from build123d import *

# Parameters (mm, degrees)
SKETCH_1_R      = 16.2
SKETCH_1_R_2    = 14.6
EXTRUDE_1_DEPTH = 2.5
SKETCH_3_R      = 1
FILLET_1_R      = 1


with BuildPart() as part:
    # 草图1 → 凸台-拉伸1 (new body, symmetric)
    with BuildSketch(Plane.XY):
        Circle(SKETCH_1_R)
        Circle(SKETCH_1_R_2, mode=Mode.SUBTRACT)
    extrude(amount=EXTRUDE_1_DEPTH, both=True)

    # 草图3 → 切除-旋转1 (revolve, cut)
    with BuildSketch(Plane(origin=(0, 0, 0), x_dir=(1, 0, 0), z_dir=(0, 1, 0))):
        with Locations((-14.1, 0)):
            Circle(SKETCH_3_R)
    revolve(axis=Axis((0, 0, 2.5), (0, 0, -1)), mode=Mode.SUBTRACT)

    # 圆角1
    fillet_1_edges = [part.edges().sort_by_distance(p)[0] for p in [
        (0, 14.6, 0.866025404),
        (0, -14.6, -0.866025404),
    ]]
    fillet(fillet_1_edges, radius=FILLET_1_R)


solid = part.part
For this review, take the finished solid that the model builds, in its own axes (mm). Give positions to 0.01 mm unless a question says otherwise; leave off trailing zeros. Order: outer loops, then holes, each group sorted by start corner. A loop starts at its lowest first (then second) coordinate and runs counter-clockwise, first axis right, second up. Notation, with made-up numbers: M -3.75,-7.5 L 38.25,-7.5 A26 ccw 38.25,16.5 Z; hole C 43,-4 d3. An arc over 180 degrees is marked long. Answer in a Markdown table with one row per item. Add a question column.
(1) Mouldability with a two-part tool opening along Y and no side actions: class faces 1 (the face through (-8.5, 12.1, -2.5)), 2 (the face through (-3.512, -15.815, 0.035)), 3 (the face through (13.926, 4.385, 1.903)) as +Y half, -Y half, draft (parallel to the pull), parting line (faces both ways), or undercut.
(2) Consider section A-A on z = 1.85. State the section outline as (x, y) points, and give its area (3 significant figures).
(3) Wall thickness on probe 1 along Y at (x, z) = (0, -1.65); probe 2 along X at (y, z) = (6, 0.35); probe 3 along X at (y, z) = (5, -0.05): over which ranges is each line inside the solid? List them lowest first. Write a range as [from, to].
(4) For pin 1 (1 mm diameter, centred on y = -5.5, z = 0.5, fed in from +X); pin 2 (1.5 mm diameter, centred on x = 2.5, z = 0, fed in from -Y); pin 3 (1.5 mm diameter, centred on y = 12.5, z = 0.5, fed in from +X), all flat-tipped, find the tip position at first contact; note any pin that passes through.
Evaluation:
| question | item | result |
|---|---|---|
| 1 | face 1 | draft |
| 1 | face 2 | parting line |
| 1 | face 3 | undercut |
| 2 | outline | C 0,0 d32.4; hole C 0,0 d29.2 |
| 2 | area | 155 mm^2 |
| 3 | probe 1 | y = [-16.2, -14.6], [14.6, 16.2] |
| 3 | probe 2 | x = [-15.05, -13.79], [13.79, 15.05] |
| 3 | probe 3 | x = [-15.41, -14.25], [14.25, 15.41] |
| 4 | pin 1 | stops at x = 15.41 |
| 4 | pin 2 | stops at y = -16.11 |
| 4 | pin 3 | stops at x = 11.15 |
